Print and shaded views of the part. All mm, measured from the part's lowest x, y and z. A direction names the side the tool comes from. Coordinates: 2 decimals unless noted, no trailing zeros. Order: outer loops, then holes, each group sorted by start corner. A loop starts at its lowest first (then second) coordinate and runs counter-clockwise, first axis right, second up. Notation, with made-up numbers: M 66,79 L 123,79 A28 cw 123,111 Z; hole C -11,25.5 d8. An arc over 180 degrees is marked long. Return JSON: item names as keys, results as strings.
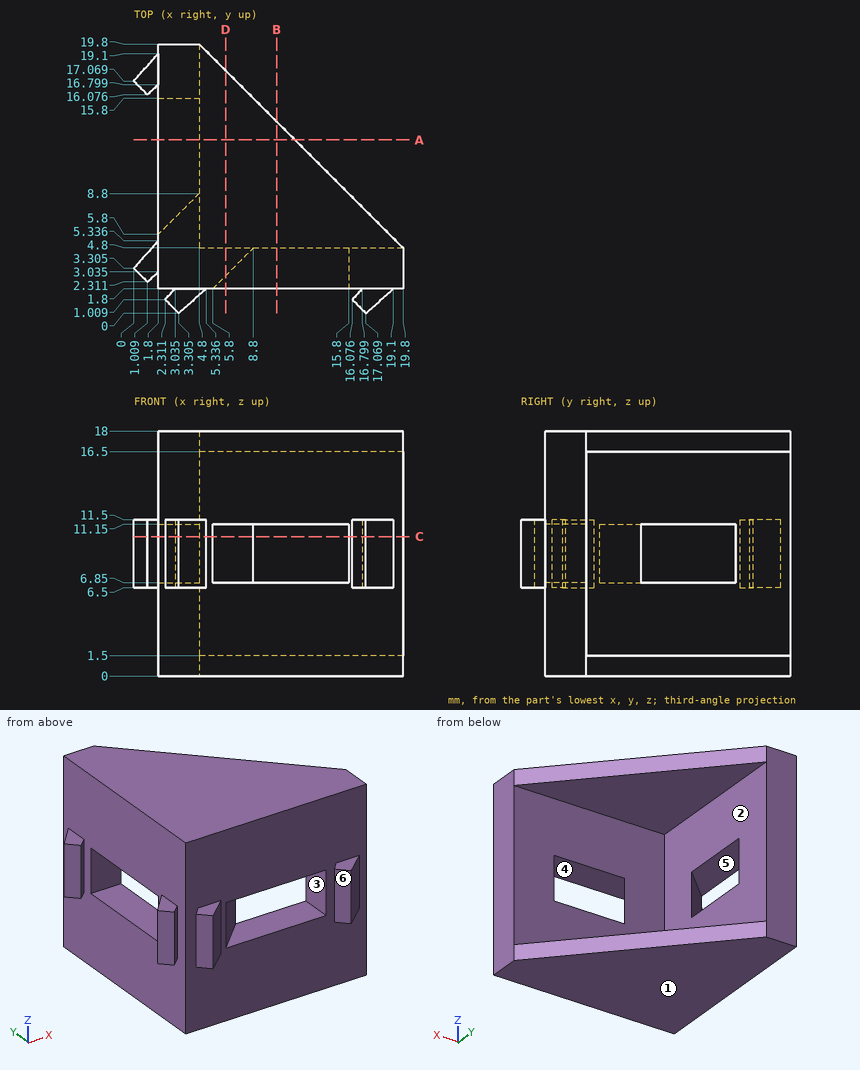
Item 1: Saw through at C-C (z = 10.25). Count the separate pieces of the cut face and the enclosed holes in it.
Check result:
{"separate pieces": "3", "enclosed holes": "0"}
Item 2: Wall check: line 1 (Z direction, x = 15.25, y = 5.25); line 2 (Y direction, x = 2.25, z = 4.5); line 3 (X direction, y = 7.5, z = 16.25). Give the ranges that are in metal, low to high.
Check result:
{"line 1": "z = 0 to 1.5, 16.5 to 18", "line 2": "y = 1.8 to 19.8", "line 3": "x = 1.8 to 4.8"}
Item 3: Drop flat-ended pins along their axis: pin 1 Ø10 at (y, z) = (11.5, 8.5) entering from +X; pin 2 Ø1.4 at (x, y) = (17.5, 1) entering from -Z; pin 3 Ø2 at (x, z) = (10, 4) entering from -Y. Give the stop position or say it passes through.
Check result:
{"pin 1": "stops at x = 4.8", "pin 2": "stops at z = 6.5", "pin 3": "stops at y = 1.8"}
Item 4: Saw through at B-B (x = 10.5). Write the cut outline in (y, z).
Check result:
{"outline": "M 1.8,0 L 14.1,0 L 14.1,1.5 L 4.8,1.5 L 4.8,6.85 L 1.8,6.85 Z; M 1.8,11.15 L 4.8,11.15 L 4.8,16.5 L 14.1,16.5 L 14.1,18 L 1.8,18 Z"}
Item 5: Pull direction X, two halves, no side cores. Call the marked faces 1, 2 and 3: +X half, -X half, draft (parallel to the pull), parting line (faces both ways), or undercut.
Check result:
{"face 1": "draft", "face 2": "+X half", "face 3": "undercut"}
Item 6: Saw through at D-D (x = 6.75). Write the cut outline in (y, z).
Check result:
{"outline": "M 1.8,0 L 17.85,0 L 17.85,1.5 L 4.8,1.5 L 4.8,16.5 L 17.85,16.5 L 17.85,18 L 1.8,18 L 1.8,11.15 L 2.75,11.15 L 2.75,6.85 L 1.8,6.85 Z"}
Item 7: 3-axis set-ups, long thin cutter, end or side, ignore diameter. For the marked faces 4, 5 and 6: which of +Z, -Z, +X, -X, +Y, -Y reach the whole face in a straight line?
Check result:
{"face 4": "-Y", "face 5": "-X", "face 6": "+Z, -Z, -Y"}
Item 8: Saw through at A-A (y = 12.75). Write the cut outline in (x, z).
Check result:
{"outline": "M 1.8,0 L 11.85,0 L 11.85,1.5 L 4.8,1.5 L 4.8,6.85 L 1.8,6.85 Z; M 1.8,11.15 L 4.8,11.15 L 4.8,16.5 L 11.85,16.5 L 11.85,18 L 1.8,18 Z"}
